```python
from build123d import *
from build123d.topology import SkipClean

# Parameters (mm, degrees)
CROQUIS1_W                   = 11
CROQUIS1_H                   = 14
CHAFL_N1_SIZE                = 1
SALIENTE_EXTRUIR1_REACH      = 31.086
SALIENTE_EXTRUIR1_END_RADIUS = 11
CROQUIS2_R                   = 6
MATRIZC1_COUNT               = 4
MATRIZC4_COUNT               = 4


with BuildPart() as part:
    # Croquis1 → Revolución1 (revolve)
    with BuildSketch(Plane(origin=(0, 0, 0), x_dir=(0, 0, -1), z_dir=(1, 0, 0))):
        with Locations((5.5, 7)):
            Rectangle(CROQUIS1_W, CROQUIS1_H)
    revolve(axis=Axis((0, 0, 0), (0, 1, 0)))

    # Chaflán1
    chafl_n1_edges = [part.edges().sort_by_distance(p)[0] for p in [
        (0, 0, 11),
        (0, 14, 11),
    ]]
    chamfer(chafl_n1_edges, length=CHAFL_N1_SIZE)

    # Saliente-Extruir1: up to this cylinder (the profile starts outside it)
    with SkipClean():  # the faces are left unmerged after this step: merging them gives an invalid solid
        saliente_extruir1_end = Plane(origin=(0, 7, 0), z_dir=(0, -1, 0)) * Cylinder(SALIENTE_EXTRUIR1_END_RADIUS, 85.172, mode=Mode.PRIVATE)
        # Croquis2 → Saliente-Extruir1 (add, up to the surface)
        with BuildSketch(Plane.XY.offset(12), mode=Mode.PRIVATE) as saliente_extruir1_sk1:
            with Locations((0, 7)):
                Circle(CROQUIS2_R)
        saliente_extruir1_tool1 = extrude(saliente_extruir1_sk1.sketch, amount=-SALIENTE_EXTRUIR1_REACH, mode=Mode.PRIVATE) - saliente_extruir1_end
        saliente_extruir1 = saliente_extruir1_tool1.solids().sort_by_distance((0, 7, 12))[0]
        add(saliente_extruir1)

    # MatrizC1: Saliente-Extruir1 ×4 about axis
    matrizc1_axis = Axis((0, 0, 0), (0, 1, 0))
    for i in range(1, MATRIZC1_COUNT):
        add(saliente_extruir1.rotate(matrizc1_axis, i * 360 / MATRIZC1_COUNT))

    # Croquis4 → Cortar-Revolución1 (revolve, cut)
    with BuildSketch(Plane.XY):
        Polygon((3.5, 7), (12, 7), (12, 3), (5, 3), align=None)
    cortar_revoluci_n1 = revolve(axis=Axis((3.5, 7, 0), (1, 0, 0)), mode=Mode.SUBTRACT)

    # MatrizC4: Cortar-Revolución1 ×4 about axis
    matrizc4_axis = Axis((0, 14, 0), (0, 1, 0))
    for i in range(1, MATRIZC4_COUNT):
        add(cortar_revoluci_n1.rotate(matrizc4_axis, i * 360 / MATRIZC4_COUNT), mode=Mode.SUBTRACT)


solid = part.part
```
Geometry check sheet. Reference: the model listing, model coordinates, mm. A direction names the side the tool comes from. Round coordinates to 2 decimals unless told otherwise and drop trailing zeros. Order: outer loops, then holes, each group sorted by start corner. A loop starts at its lowest first (then second) coordinate and runs counter-clockwise, first axis right, second up. Notation, with made-up numbers: M 37,48 L 89,48 A16 ccw 89,78 Z; hole C 73.25,-10.5 d6. An arc over 180 degrees is marked long. Write item = value, one per line.
Q1. Set-up check for faces 4 (the cylindrical face through (0, 11, 8)), 5 (the flat face through (-12, 8.42, 3.92)), 6 (the cylindrical face through (4.76, 3.35, -10.94)): record each of +Z, -Z, +X, -X, +Y, -Y from which the full face is reachable in a straight line by a thin tool's end or side.
Answer block:
face_4 = +Z
face_5 = +Z, -Z, -X, +Y, -Y
face_6 = -Z
Q2. Section check A-A (y = 2.5). Enter the section's corners in (x, z).
Answer block:
outline = M -12,-3.97 L -10.26,-3.97 A11 ccw -3.97,-10.26 L -3.97,-12 L 3.97,-12 L 3.97,-10.26 A11 ccw 10.26,-3.97 L 12,-3.97 L 12,3.97 L 10.26,3.97 A11 ccw 3.97,10.26 L 3.97,12 L -3.97,12 L -3.97,10.26 A11 ccw -10.26,3.97 L -12,3.97 Z
Q3. Scan lines: line 1 (X direction, y = 7.25, z = 10); line 2 (Y direction, x = 3, z = -10.5); line 3 (Z direction, x = -9, y = 7). Record each from-to range of solid material in increasing order.
Answer block:
line_1 = -5.99 to -3.99, 3.99 to 5.99
line_2 = 0.92 to 4.35, 9.65 to 13.08
line_3 = -6.32 to -4, 4 to 6.32
Q4. Release check for a two-part mould opening along Z. For faces 1 (the conical face through (-3.57, 7.19, 0.01)), 2 (the flat face through (12, 8.42, -3.92)), 3 (the conical face through (-0.01, 7.19, -3.57)) record: released by +Z, released by -Z, zero draft, split by the parting line, or undercut.
Answer block:
face_1 = undercut
face_2 = zero draft
face_3 = released by -Z
Q5. Depth check by flat-ended pin: pin 1 Ø5 at (y, z) = (7, 0) entering from -X; pin 2 Ø8 at (y, z) = (12.5, 8) entering from +X; pin 3 Ø7 at (x, y) = (0, 7) entering from -Z; pin 4 Ø7 at (x, y) = (0, 7) entering from +Z. Enter the tip coordinate at first touch or a pass-through.
Answer block:
pin_1 = -4.44
pin_2 = 12
pin_3 = -4.81
pin_4 = 4.81
